Autodesk Inventor part; units mm, degrees
ref_plane "YZ Plane" through (0, 0, 0) normal (1, 0, 0) x (0, 1, 0)
ref_plane "XZ Plane" through (0, 0, 0) normal (0, 1, 0) x (-1, 0, 0)
ref_plane "XY Plane" through (0, 0, 0) normal (0, 0, 1) x (1, 0, 0)
sketch "Sketch1" plane through (0, 0, 0) normal (0, 0, 1) x (1, 0, 0)
  line L0 (-850, -500) -> (850, -500)
  line L1 (850, -500) -> (850, 500)
  line L2 (850, 500) -> (-850, 500)
  line L3 (-850, 500) -> (-850, -500)
  line L4 (-850, -500) -> (850, 500) construction
  line L5 (850, -500) -> (-850, 500) construction
  point P0 (0, 0)
  dimension "d0" = 1700
  dimension "d1" = 1000
extrude "Extrusion1" add sketch "Sketch1" along normal blind 100
sketch "Sketch2" plane through (0, 0, 0) normal (0, 0, -1) x (-1, 0, 0)
  line L0 (-817.5, 467.5) -> (817.5, 467.5)
  line L1 (817.5, 467.5) -> (817.5, -467.5)
  line L2 (817.5, -467.5) -> (-817.5, -467.5)
  line L3 (-817.5, -467.5) -> (-817.5, 467.5)
  line L4 (-817.5, 467.5) -> (817.5, -467.5) construction
  line L5 (817.5, 467.5) -> (-817.5, -467.5) construction
  line L6 (850, 500) -> (850, -500)
  line L7 (850, -500) -> (-850, -500)
  point P0 (0, 0)
  dimension "d4" = 32.5
  dimension "d5" = 32.5
extrude "Extrusion2" cut sketch "Sketch2" against normal blind 60
sketch "Sketch3" plane through (850, -500, 0) normal (1, 0, 0) x (0, 0, -1)
  circle A0 centre (-50, 250) radius 30
  circle A1 centre (-50, 750) radius 30
  point P0 (0, 500)
  dimension "d8" = 60
  dimension "d9" = 60
extrude "Extrusion3" add sketch "Sketch3" along normal blind 350 contours A0
sketch "Sketch4" plane through (850, -500, 0) normal (1, 0, 0) x (0, 0, -1)
  circle A0 centre (-50, 750) radius 30
  point P0 (0, 500)
  dimension "d12" = 60
extrude "Extrusion4" add sketch "Sketch4" along normal blind 350
chamfer "Chamfer1" distance 10 angle 45 1 edges at (1200, -250, 80)
chamfer "Chamfer2" distance 10 angle 45 1 edges at (1200, 250, 80)
properties part number "top"
Check sheet for the modelled part. Datum: model origin and axes. Units: mm. A direction names the side the tool comes from. Give positions to 0.01 mm unless a question says otherwise; leave off trailing zeros. Order: outer loops, then holes, each group sorted by start corner. A loop starts at its lowest first (then second) coordinate and runs counter-clockwise, first axis right, second up. Notation, with made-up numbers: M 45,35 L 84,35 A9 ccw 84,39 Z; hole C 1.25,-16.5 d7. An arc over 180 degrees is marked long. Answer as CSV lines item,"result". Start each with the question number.
Item 1: Thickness scan on line 1 (X direction, y = -242, z = 45); line 2 (X direction, y = -14.5, z = 36); line 3 (Y direction, x = -268, z = 56.5). Record the ranges inside material, lowest first. Write a range as [from, to].
Item 2: Gauge pin test, flat ends, axial feed: P1, Ø3, axis at x = -218, y = -85.5, coming from the -Z side; P2, Ø8, axis at y = 299.5, z = 15, coming from the +X side. Record the tip position at first contact, or that the pin passes through.
Item 3: Cross-section at B-B on x = 752.5. Enter the section's corners in (y, z).
Item 4: Cross-section at A-A on y = 250. Enter the section's corners in (x, z).
Item 5: Mould release check, pull along Y, two halves, no side actions. Record for faces 4 (the face through (-12, -500, 49)), 5 (the face through (-11, -467.5, 30)), 6 (the face through (1200, -250, 50)): +Y half, -Y half, draft (parallel to the pull), parting line (faces both ways), or undercut.
Item 6: Tool access check on faces 1 (the face through (-256, -479, 0)), 2 (the face through (1017.62, -279.745, 53.905)), 3 (the face through (817.5, -7, 30)). Record the directions out of +Z, -Z, +X, -X, +Y, -Y that give a thin tool (end or side, any length) a straight path to the whole face; none if there is none.
Item 7: Cross-section at C-C on y = -419.5. Enter the section's corners in (x, z).
Established:
1,line 1,"x = [-850, -817.5], [817.5, 1200]"
1,line 2,"x = [-850, -817.5], [817.5, 850]"
1,line 3,"y = [-500, -467.5], [467.5, 500]"
2,P1,"stops at z = 60"
2,P2,"stops at x = 850"
3,outline,"M -500,0 L -467.5,0 L -467.5,60 L 467.5,60 L 467.5,0 L 500,0 L 500,100 L -500,100 Z"
4,outline,"M -850,0 L -817.5,0 L -817.5,60 L 817.5,60 L 817.5,0 L 850,0 L 850,20 L 1190,20 L 1200,30 L 1200,70 L 1190,80 L 850,80 L 850,100 L -850,100 Z"
5,face 4,"-Y half"
5,face 5,"undercut"
5,face 6,"draft"
6,face 1,"-Z, +X, -X, +Y, -Y"
6,face 2,"+X"
6,face 3,"-Z"
7,outline,"M -850,0 L -817.5,0 L -817.5,60 L 817.5,60 L 817.5,0 L 850,0 L 850,100 L -850,100 Z"
